```python
from build123d import *

# Parameters (mm, degrees)
BOSS_EXTRUDE1_DEPTH          = 32
SKETCH2_R                    = 15
CUT_EXTRUDE1_DEPTH           = 1
SKETCH3_R                    = 10
SKETCH3_R_2                  = 5
BOSS_EXTRUDE2_DEPTH          = 2
BOSS_EXTRUDE3_DEPTH          = 32
F_3_0_3_DIAMETER_HOLE1_D     = 3
F_3_0_3_DIAMETER_HOLE1_DEPTH = 5
F_3_0_3_DIAMETER_HOLE1_TIP   = 0.901290929


with BuildPart() as part:
    # Sketch1 → Boss-Extrude1 (new body)
    with BuildSketch(Plane(origin=(0, 0, 0), x_dir=(1, 0, 0), z_dir=(0, 1, 0))):
        Polygon((-20.5, 18.5), (-18.5, 20.5), (18.5, 20.5), (20.5, 18.5), (20.5, -18.5), (18.5, -20.5), (-18.5, -20.5), (-20.5, -18.5), align=None)
    extrude(amount=BOSS_EXTRUDE1_DEPTH)

    # Sketch2 → Cut-Extrude1 (cut)
    with BuildSketch(Plane(origin=(0, 32, 0), x_dir=(-1, 0, 0), z_dir=(0, 1, 0))):
        with Locations(Location((0, 0, 0), (0, 0, 90))):
            Circle(SKETCH2_R)
    extrude(amount=-CUT_EXTRUDE1_DEPTH, mode=Mode.SUBTRACT)

    # Sketch3 → Boss-Extrude2 (add)
    with BuildSketch(Plane(origin=(0, 31, 0), x_dir=(1, 0, 0), z_dir=(0, 1, 0))):
        with Locations(Location((0, 0, 0), (0, 0, 270))):
            Circle(SKETCH3_R)
        with Locations(Location((0, 0, 0), (0, 0, 270))):
            Circle(SKETCH3_R_2, mode=Mode.SUBTRACT)
    extrude(amount=BOSS_EXTRUDE2_DEPTH)

    # Sketch4 → Boss-Extrude3 (add)
    with BuildSketch(Plane(origin=(0, 31, 0), x_dir=(1, 0, 0), z_dir=(0, 1, 0))):
        with BuildLine():
            Line((-1.470984161, 2.175359116), (1.470984161, 2.175359116))
            ThreePointArc((1.470984161, 2.175359116), (0, -2.626020123), (-1.470984161, 2.175359116))
        make_face()
    extrude(amount=BOSS_EXTRUDE3_DEPTH)

    # 3.0 _3_ Diameter Hole1
    with Locations(Plane(origin=(0, 32, 0), x_dir=(-1, 0, 0), z_dir=(0, 1, 0))):
        with Locations((-15.5, -15.5), (15.5, -15.5), (15.5, 15.5), (-15.5, 15.5)):
            Hole(F_3_0_3_DIAMETER_HOLE1_D / 2, depth=F_3_0_3_DIAMETER_HOLE1_DEPTH)
            with Locations((0, 0, -(F_3_0_3_DIAMETER_HOLE1_DEPTH + F_3_0_3_DIAMETER_HOLE1_TIP / 2))):  # 118° drill point
                Cone(0, F_3_0_3_DIAMETER_HOLE1_D / 2, F_3_0_3_DIAMETER_HOLE1_TIP, mode=Mode.SUBTRACT)


solid = part.part
```
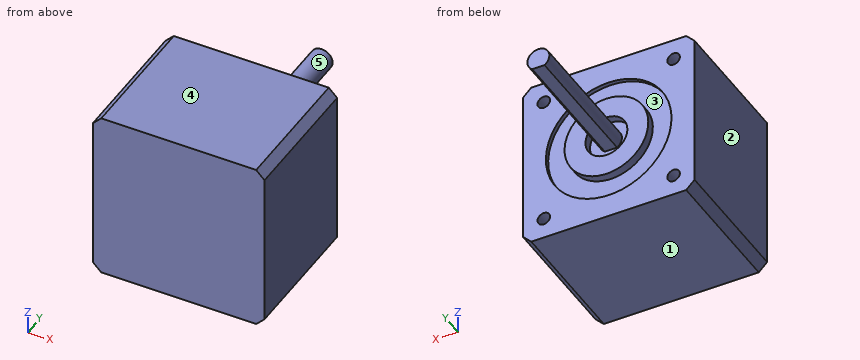
Input: part model. Units: mm. Frame: model coordinates. Face numbers are marked on the shaded views. A direction names the side the tool comes from. Round coordinates to 2 decimals unless told otherwise and drop trailing zeros. Loops run counter-clockwise (first coordinate to the right, second up) from the corner with the lowest first, then second, coordinate; pieces in that order, holes last. Notation, with made-up numbers: (-32.75, 38.5) -> (-22.75, 38.5) arc R24 ccw to (-22.75, 77.5) -> close; hole circle Ø3 at (78, 79). An arc over 180 degrees is marked (long way). Write each question's results on one line, items separated by ' | '.
1. Section A-A (x = 12). Return loops of the section in (y, z), and give its area (3 significant figures).
Geometry results:
outline: (0, -20.5) -> (32, -20.5) -> (32, -9) -> (31, -9) -> (31, 9) -> (32, 9) -> (32, 20.5) -> (0, 20.5) -> close | area: 1,290 mm2
2. Ray query, line 1 (X direction, y = 28.1, z = -15.5); line 2 (X direction, y = 31.6, z = 0). Return the intervals inside material, ascending. Write a range as from..to.
Geometry results:
line 1: -20.5..-17, -14..14, 17..20.5 | line 2: -20.5..-15, -10..-5, -2.63..2.63, 5..10, 15..20.5
3. Section C-C (z = -7). Return loops of the section in (x, y), and give its area (3 significant figures).
Geometry results:
outline: (-20.5, 0) -> (20.5, 0) -> (20.5, 32) -> (13.27, 32) -> (13.27, 31) -> (7.14, 31) -> (7.14, 33) -> (-7.14, 33) -> (-7.14, 31) -> (-13.27, 31) -> (-13.27, 32) -> (-20.5, 32) -> close | area: 1,310 mm2
4. Mould query, pull axis Z, two halves, no side actions, for the marked faces 1, 2 and 3. Classes: +Z half, -Z half, draft (parallel to the pull), parting line (faces both ways), or undercut.
Geometry results:
face 1: -Z half | face 2: draft | face 3: undercut
5. Section D-D (z = 8). Return loops of the section in (x, y).
Geometry results:
outline: (-20.5, 0) -> (20.5, 0) -> (20.5, 32) -> (12.69, 32) -> (12.69, 31) -> (6, 31) -> (6, 33) -> (-6, 33) -> (-6, 31) -> (-12.69, 31) -> (-12.69, 32) -> (-20.5, 32) -> close
6. Set-up query: the marked faces 4 and 5. Return all of +Z, -Z, +X, -X, +Y, -Y with unobstructed straight access to the full face (end or side cutting, diameter ignored); none if empty.
Geometry results:
face 4: +Z, +X, -X, +Y, -Y | face 5: +Y
7. Section B-B (z = 0). Return loops of the section in (x, y), and give its area (3 significant figures).
Geometry results:
outline: (-20.5, 0) -> (20.5, 0) -> (20.5, 32) -> (15, 32) -> (15, 31) -> (10, 31) -> (10, 33) -> (5, 33) -> (5, 31) -> (2.63, 31) -> (2.63, 63) -> (-2.63, 63) -> (-2.63, 31) -> (-5, 31) -> (-5, 33) -> (-10, 33) -> (-10, 31) -> (-15, 31) -> (-15, 32) -> (-20.5, 32) -> close | area: 1,470 mm2
8. First-contact query: P1, Ø3.5, axis at x = -15.5, z = -15.5, coming from the +Y side; P2, Ø5, axis at y = 40, z = -2.5, coming from the -X side; P3, Ø5, axis at y = 45, z = -2.5, coming from the +X side. Flat tips, straight axial feed; report the tip coordinate or a pass-through.
Geometry results:
P1: y = 32 | P2: x = -2.63 | P3: x = 2.63
